```python
from build123d import *

# Parameters (mm, degrees)
CYLINDER002_R     = 10.8
CYLINDER002_DEPTH = 3
CYLINDER004_R     = 16.7
CYLINDER004_DEPTH = 3


with BuildPart() as cylinder002:
    # Cylinder002 → Cylinder002 (new body)
    with BuildSketch(Plane.XY.offset(57)):
        Circle(CYLINDER002_R)
    extrude(amount=CYLINDER002_DEPTH)


with BuildPart() as obj1:
    # Cylinder004 → Cylinder004 (new body)
    with BuildSketch(Plane.XY.offset(57)):
        Circle(CYLINDER004_R)
    extrude(amount=CYLINDER004_DEPTH)

    # Cut: cut Cylinder002
    add(cylinder002.part, mode=Mode.SUBTRACT)


solid = obj1.part
```
Verification items for the finished model (mm, model axes). Give positions to 0.01 mm unless a question says otherwise; leave off trailing zeros. Write each loop counter-clockwise with the first axis right and the second up, starting at its lowest first coordinate (ties: lowest second). Pieces come first, ordered by that corner, then holes. Notation, with made-up numbers: M 74,9 L 119,9 A13 cw 119,19 Z; hole C 59,78 d1. An arc over 180 degrees is marked long. One line per question, with ' | ' between items.
1) Section check C-C on z = 58.15. Enter the section's corners in (x, y).
Result:
outline: C 0,0 d33.4; hole C 0,0 d21.6
2) Mould release check, pull along X, two halves, no side actions. Record for faces 1 (the flat face through (0, -11, 57)), 2 (the cylindrical face through (15.929, 5.016, 58.479)), 3 (the cylindrical face through (-2.341, -10.543, 58.479)): released by +X, released by -X, zero draft, split by the parting line, or undercut.
Result:
face 1: zero draft | face 2: split by the parting line | face 3: undercut
3) Section check A-A on x = 0. Enter the section's corners in (y, z), plus the area to 3 significant figures.
Result:
outline: M -16.7,57 L -10.8,57 L -10.8,60 L -16.7,60 Z; M 10.8,57 L 16.7,57 L 16.7,60 L 10.8,60 Z | area: 35.4 mm2
4) Gauge pin test, flat end, axial feed: pin 1 Ø1.5 at (y, z) = (-4.5, 57.5) entering from +X. Record the tip position at first contact, or that the pin passes through.
Result:
pin 1: stops at x = 16.27
5) Section check D-D on y = -13. Enter the section's corners in (x, z), plus the area to 3 significant figures.
Result:
outline: M -10.48,57 L 10.48,57 L 10.48,60 L -10.48,60 Z | area: 62.9 mm2
6) Thickness scan on line 1 along Y through (x, z) = (0, 58.95); line 2 along Y through (x, z) = (-6, 59.45); line 3 along X through (y, z) = (-4, 57.45). Record the ranges inside material, lowest first. Write a range as [from, to].
Result:
line 1: y = [-16.7, -10.8], [10.8, 16.7] | line 2: y = [-15.58, -8.98], [8.98, 15.58] | line 3: x = [-16.21, -10.03], [10.03, 16.21]
